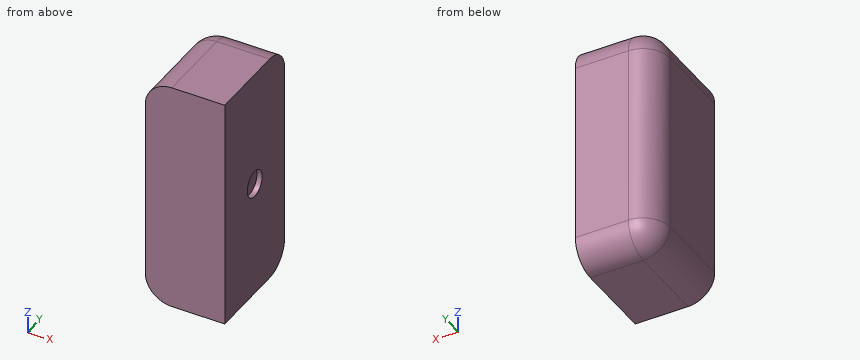
from build123d import *

# Parameters (mm, degrees)
SKETCH1_W           = 30
SKETCH1_H           = 88.4
BOSS_EXTRUDE1_DEPTH = 40
FILLET1_R           = 10
SKETCH2_R           = 5
CUT_EXTRUDE1_DEPTH  = 2


with BuildPart() as part:
    # Sketch1 → Boss-Extrude1 (new body)
    with BuildSketch(Plane(origin=(0, 0, 0), x_dir=(1, 0, 0), z_dir=(0, 1, 0))):
        with Locations((15, 44.2)):
            Rectangle(SKETCH1_W, SKETCH1_H)
    extrude(amount=BOSS_EXTRUDE1_DEPTH)

    # Fillet1
    fillet1_edges = [part.edges().sort_by_distance(p)[0] for p in [
        (15, 40, -88.4),
        (0, 40, -44.2),
        (0, 20, -88.4),
        (0, 20, 0),
        (15, 40, 0),
    ]]
    fillet(fillet1_edges, radius=FILLET1_R)

    # Sketch2 → Cut-Extrude1 (cut)
    with BuildSketch(Plane(origin=(30, 0, 0), x_dir=(0, 0, -1), z_dir=(1, 0, 0))):
        with Locations((44.2, 20)):
            Circle(SKETCH2_R)
    extrude(amount=-CUT_EXTRUDE1_DEPTH, mode=Mode.SUBTRACT)


solid = part.part
Source: CAD feature listing. Evaluate the final solid. Frame: model axes, mm. Coordinates: 2 decimals unless noted, no trailing zeros. Loops run counter-clockwise (first coordinate to the right, second up) from the corner with the lowest first, then second, coordinate; pieces in that order, holes last. Notation, with made-up numbers: (63, 50.5) - (69, 50.5) arc R18 cw to (69, 73.5) - close; hole circle Ø11 at (30.25, 11.5). An arc over 180 degrees is marked (long way). One line per item, written item: value. Start each with the question number.
1. Contact query for a flat-ended pin moving along its axis: P1, Ø3, axis at y = 19.5, z = -45, coming from the +X side. Output: stop coordinate, or through.
2. Section D-D (z = -44.2). Return the cut outline in (x, y), and give its area (3 significant figures).
3. Section C-C (x = 2). Return the cut outline in (y, z).
4. Section A-A (z = -70.5). Return the cut outline in (x, y), and give its area (3 significant figures).
5. Ray query, L1, parallel to Y at x = 29.55, z = -44.2; L2, parallel to X at y = 21, z = -49; L3, parallel to Y at x = 25, z = -5. Return the intervals inside material, ascending.
6. Section B-B (y = 20). Return the cut outline in (x, z).
Verdict:
1. P1: stops at x = 28
2. outline: (0, 0) - (30, 0) - (30, 15) - (28, 15) - (28, 25) - (30, 25) - (30, 40) - (10, 40) arc R10 ccw to (0, 30) - close
2. area: 1,160 mm2
3. outline: (0, -84.4) - (30, -84.4) arc R6 ccw to (36, -78.4) - (36, -10) arc R6 ccw to (30, -4) - (0, -4) - close
4. outline: (0, 0) - (30, 0) - (30, 40) - (10, 40) arc R10 ccw to (0, 30) - close
4. area: 1,180 mm2
5. L1: y = 0 to 15, 25 to 40
5. L2: x = 0 to 28
5. L3: y = 0 to 38.66
6. outline: (0, -78.4) arc R10 ccw to (10, -88.4) - (30, -88.4) - (30, -49.2) - (28, -49.2) - (28, -39.2) - (30, -39.2) - (30, 0) - (10, 0) arc R10 ccw to (0, -10) - close
